The model under review builds one solid part; all positions refer to its coordinate system, in mm. Coordinates: 2 decimals unless noted, no trailing zeros. Order: outer loops, then holes, each group sorted by start corner. A loop starts at its lowest first (then second) coordinate and runs counter-clockwise, first axis right, second up. Notation, with made-up numbers: (11.5, 32.5) -> (56.5, 32.5) arc R23 ccw to (56.5, 54.5) -> close; hole circle Ø9 at (81.5, -0.75). An arc over 180 degrees is marked (long way). Use CSV: the item, a comma, the result in double quotes. Start each with the question number.
```python
from build123d import *

# Parameters (mm, degrees)
SKETCH1_R           = 57
BOSS_EXTRUDE1_DEPTH = 2.5


with BuildPart() as part:
    # Sketch1 → Boss-Extrude1 (new, symmetric)
    with BuildSketch(Plane(origin=(0, 0, 0), x_dir=(1, 0, 0), z_dir=(0, 1, 0))):
        with Locations(Location((0, 0, 0), (0, 0, 270))):
            Circle(SKETCH1_R)
        with BuildLine():
            Line((14.789875777, 42.235317857), (16.959294472, 46.740162197))
            Line((16.959294472, 46.740162197), (25.968983151, 42.401324806))
            Line((25.968983151, 42.401324806), (23.799564456, 37.896480466))
            ThreePointArc((23.799564456, 37.896480466), (27.901168633, 34.98695884), (31.65043527, 31.635619912))
            Line((31.65043527, 31.635619912), (35.559592682, 34.753068922))
            Line((35.559592682, 34.753068922), (41.7944907, 26.934754097))
            Line((41.7944907, 26.934754097), (37.885333288, 23.817305088))
            ThreePointArc((37.885333288, 23.817305088), (40.318356839, 19.416297326), (42.24223789, 14.770099458))
            Line((42.24223789, 14.770099458), (47.116877451, 15.882704128))
            Line((47.116877451, 15.882704128), (49.342086791, 6.133425006))
            Line((49.342086791, 6.133425006), (44.46744723, 5.020820337))
            ThreePointArc((44.46744723, 5.020820337), (44.679305968, 2.514382276), (44.75, 0))
            ThreePointArc((44.75, 0), (44.679305968, -2.514382276), (44.46744723, -5.020820337))
            Line((44.46744723, -5.020820337), (49.342086791, -6.133425006))
            Line((49.342086791, -6.133425006), (47.116877451, -15.882704128))
            Line((47.116877451, -15.882704128), (42.24223789, -14.770099458))
            ThreePointArc((42.24223789, -14.770099458), (40.318356839, -19.416297326), (37.885333288, -23.817305088))
            Line((37.885333288, -23.817305088), (41.7944907, -26.934754097))
            Line((41.7944907, -26.934754097), (35.559592682, -34.753068922))
            Line((35.559592682, -34.753068922), (31.65043527, -31.635619912))
            ThreePointArc((31.65043527, -31.635619912), (27.901168633, -34.98695884), (23.799564456, -37.896480466))
            Line((23.799564456, -37.896480466), (25.968983151, -42.401324806))
            Line((25.968983151, -42.401324806), (16.959294472, -46.740162197))
            Line((16.959294472, -46.740162197), (14.789875777, -42.235317857))
            ThreePointArc((14.789875777, -42.235317857), (9.957811795, -43.62802407), (5, -44.469793118))
            Line((5, -44.469793118), (5, -49.469793118))
            Line((5, -49.469793118), (-5, -49.469793118))
            Line((-5, -49.469793118), (-5, -44.469793118))
            ThreePointArc((-5, -44.469793118), (-9.957811795, -43.62802407), (-14.789875777, -42.235317857))
            Line((-14.789875777, -42.235317857), (-16.959294472, -46.740162197))
            Line((-16.959294472, -46.740162197), (-25.968983151, -42.401324806))
            Line((-25.968983151, -42.401324806), (-23.799564456, -37.896480466))
            ThreePointArc((-23.799564456, -37.896480466), (-27.901168633, -34.98695884), (-31.65043527, -31.635619912))
            Line((-31.65043527, -31.635619912), (-35.559592682, -34.753068922))
            Line((-35.559592682, -34.753068922), (-41.7944907, -26.934754097))
            Line((-41.7944907, -26.934754097), (-37.885333288, -23.817305088))
            ThreePointArc((-37.885333288, -23.817305088), (-40.318356839, -19.416297326), (-42.24223789, -14.770099458))
            Line((-42.24223789, -14.770099458), (-47.116877451, -15.882704128))
            Line((-47.116877451, -15.882704128), (-49.342086791, -6.133425006))
            Line((-49.342086791, -6.133425006), (-44.46744723, -5.020820337))
            ThreePointArc((-44.46744723, -5.020820337), (-44.75, 0), (-44.46744723, 5.020820337))
            Line((-44.46744723, 5.020820337), (-49.342086791, 6.133425006))
            Line((-49.342086791, 6.133425006), (-47.116877451, 15.882704128))
            Line((-47.116877451, 15.882704128), (-42.24223789, 14.770099458))
            ThreePointArc((-42.24223789, 14.770099458), (-40.318356839, 19.416297326), (-37.885333288, 23.817305088))
            Line((-37.885333288, 23.817305088), (-41.7944907, 26.934754097))
            Line((-41.7944907, 26.934754097), (-35.559592682, 34.753068922))
            Line((-35.559592682, 34.753068922), (-31.65043527, 31.635619912))
            ThreePointArc((-31.65043527, 31.635619912), (-27.901168633, 34.98695884), (-23.799564456, 37.896480466))
            Line((-23.799564456, 37.896480466), (-25.968983151, 42.401324806))
            Line((-25.968983151, 42.401324806), (-16.959294472, 46.740162197))
            Line((-16.959294472, 46.740162197), (-14.789875777, 42.235317857))
            ThreePointArc((-14.789875777, 42.235317857), (-9.957811795, 43.62802407), (-5, 44.469793118))
            Line((-5, 44.469793118), (-5, 49.469793118))
            Line((-5, 49.469793118), (5, 49.469793118))
            Line((5, 49.469793118), (5, 44.469793118))
            ThreePointArc((5, 44.469793118), (9.957811795, 43.62802407), (14.789875777, 42.235317857))
        make_face(mode=Mode.SUBTRACT)
    extrude(amount=BOSS_EXTRUDE1_DEPTH, both=True)


solid = part.part
```
Q1. Add section A-A, the plane z = 0. State the section outline as (x, y) points, then the cut area to 4 significant figures.
Q2. Draft analysis for pull direction X (two halves, no side actions). For faces 1 (the cylindrical face through (-55.645, 0.035, -12.356)), 2 (the flat face through (-42, 2.5, 17)), 3 (the flat face through (0, 0, 49.47)), 4 (the flat face through (-24.9, 0.04, 40.18)), state which applies: +X half, -X half, draft (parallel to the pull), parting line (faces both ways), or undercut.
Q3. Clearance check with flat-ended pins moving along their axes: pin 1 Ø3 at (x, y) = (-42.5, -2) entering from -Z; pin 2 Ø1.5 at (y, z) = (1, -5.5) entering from -X; pin 3 Ø1 at (x, y) = (23, 0) entering from +Z. State where each tip first meets the part, or that it passes through.
Q4. Add section B-B, the plane x = 0. State the section outline as (y, z) points.
Q5. To check wall thickness, follow probe 1 along Z at (x, y) = (-47, -0.65); probe 2 along X at (y, z) = (1.1, -33); probe 3 along Z at (x, y) = (23, -1.6). State the ranges of each line that lie inside material, in increasing order.
Answer block:
1,outline,"(-57, -2.5) -> (-44.75, -2.5) -> (-44.75, 2.5) -> (-57, 2.5) -> close; (44.75, -2.5) -> (57, -2.5) -> (57, 2.5) -> (44.75, 2.5) -> close"
1,area,"122.5 mm²"
2,face 1,"parting line"
2,face 2,"draft"
2,face 3,"undercut"
2,face 4,"undercut"
3,pin 1,"stops at z = -39.6"
3,pin 2,"stops at x = -56.8"
3,pin 3,"stops at z = 52.37"
4,outline,"(-2.5, -57) -> (2.5, -57) -> (2.5, -49.47) -> (-2.5, -49.47) -> close; (-2.5, 49.47) -> (2.5, 49.47) -> (2.5, 57) -> (-2.5, 57) -> close"
5,probe 1,"z = -32.25 to -15.86, -5.6 to 5.6, 15.86 to 32.25"
5,probe 2,"x = -46.48 to -36.96, -33.36 to -30.23, 30.23 to 33.36, 36.96 to 46.48"
5,probe 3,"z = -52.15 to -43.83, 43.83 to 52.15"
